Input: part model. Units: mm. Frame: model coordinates. Face numbers are marked on the shaded views. Coordinates: 2 decimals unless noted, no trailing zeros. Loops run counter-clockwise (first coordinate to the right, second up) from the corner with the lowest first, then second, coordinate; pieces in that order, holes last.
(1) Contact query for flat-ended pins moving along their axis: P1, Ø3, axis at y = 1.5, z = -91, coming from the -X side; P2, Ø3, axis at x = 53, y = 0.5, coming from the +Z side; P3, Ø5, axis at x = 85, z = -66.5, coming from the -Y side. Output: stop coordinate, or through.
(2) Section B-B, the plane z = -51. Return loops of the section in (x, y).
(3) Line query: L1, parallel to Z at x = 83, y = 2.8; L2, parallel to Z at x = 81, y = 4.1; L3, parallel to X at y = 2.45, z = -59.5. Output: solid intervals per line, ascending.
(4) Section C-C, the plane x = 52. Return loops of the section in (y, z).
(5) Mould query, pull axis X, two halves, no side actions, for the marked faces 1, 2 and 3. Classes: released by +X, released by -X, zero draft, split by the parting line, or undercut.
(6) Section A-A, the plane x = 85.5. Return loops of the section in (y, z).
Autodesk Inventor part; units mm, degrees
ref_plane "YZ Plane" through (0, 0, 0) normal (1, 0, 0) x (0, 1, 0)
ref_plane "XZ Plane" through (0, 0, 0) normal (0, 1, 0) x (-1, 0, 0)
ref_plane "XY Plane" through (0, 0, 0) normal (0, 0, 1) x (1, 0, 0)
sketch "スケッチ1" plane through (0, 0, 0) normal (0, 1, 0) x (-1, 0, 0)
  line L0 (25, 0) -> (-25, 0)
  line L1 (-25, 0) -> (-25, -104.5)
  line L2 (-25, -104.5) -> (25, -104.5)
  line L3 (25, -104.5) -> (25, 0)
  circle A0 centre (0, 0) radius 25
  circle A1 centre (0, 0) radius 57 construction
  circle A2 centre (0, 0) radius 75 construction
  circle A3 centre (0, 0) radius 10.75
  circle A4 centre (-77.746127, -62.893082) radius 25
  circle A5 centre (-77.746127, -62.893082) radius 10.75
  line L4 (-77.746127, -62.893082) -> (-82.968428, -87.341549)
  line L5 (-82.968428, -87.341549) -> (-5.222301, -103.948468)
  line L6 (5.222301, -55.051532) -> (-72.523826, -38.444614)
  circle A6 centre (0, -79.5) radius 25
  circle A7 centre (0, 0) radius 82
  circle A8 centre (0, 0) radius 65
  line L7 (-48.165066, -43.647753) -> (-96.972293, -33.222313)
  line L8 (-96.972293, -33.222313) -> (-92.794452, -13.663539)
  line L9 (-92.794452, -13.663539) -> (-43.987225, -24.088979)
  line L10 (-43.987225, -24.088979) -> (-48.165066, -43.647753)
  line L11 (-96.972293, -33.222313) -> (-102.194595, -57.67078)
  point P0 (-25, -79.5)
  point P1 (-25, -48.595915)
  point P2 (-25, -60)
  point P3 (-48.165066, -43.647753)
  point P4 (-61.75052, -20.294661)
  dimension "d22" = 130
  dimension "d0" = 114
  dimension "d2" = 150
  dimension "d4" = 21.5
  dimension "d5" = 50
  dimension "d19" = 79.5
  dimension "d20" = 79.5
  dimension "d21" = 164
  dimension "d23" = 20
sketch "スケッチ1 outline for 押し出し1" plane through (0, 0, 0) normal (0, 1, 0) x (-1, 0, 0)
  arc A0 (-72.523826, -38.444614) -> (-82.968428, -87.341549) centre (-77.746127, -62.893082) ccw
  line L0 (-82.968428, -87.341549) -> (-5.222301, -103.948468)
  arc A1 (-5.222301, -103.948468) -> (-25, -79.5) centre (0, -79.5) cw
  line L1 (-25, -79.5) -> (-25, -60)
  arc A2 (-25, -60) -> (-48.165066, -43.647753) centre (0, 0) cw
  line L2 (-48.165066, -43.647753) -> (-72.523826, -38.444614)
  circle A3 centre (-77.746127, -62.893082) radius 10.75
extrude "押し出し1" add sketch "スケッチ1 outline for 押し出し1" along normal blind 5.5
fillet "フィレット1" radius 2 1 edges at (5.2223, 2.75, -103.9485)
equation "\"d20\" = d19"
properties part number "gear_plate_3" material "木材 (カエデ材)"
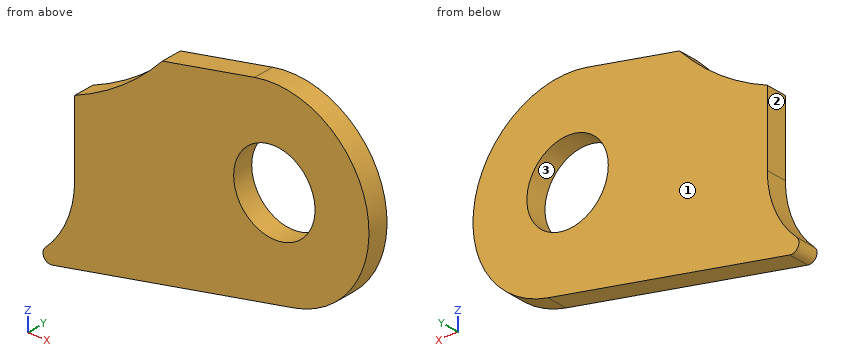
Report:
1. P1: stops at x = 21.35
1. P2: stops at z = -42.29
1. P3: passes through
2. outline: (40.3, 0) - (99.74, 0) - (99.74, 5.5) - (40.3, 5.5) - close
3. L1: z = -87.33 to -72.27, -53.51 to -38.45
3. L2: z = -87.76 to -73.14, -52.65 to -38.11
3. L3: x = 26.17 to 67.55, 87.95 to 102.51
4. outline: (0, -93.96) - (5.5, -93.96) - (5.5, -42.83) - (0, -42.83) - close
5. face 1: zero draft
5. face 2: released by -X
5. face 3: undercut
6. outline: (0, -86.66) - (5.5, -86.66) - (5.5, -70.34) - (0, -70.34) - close; (0, -55.45) - (5.5, -55.45) - (5.5, -39.13) - (0, -39.13) - close
